The drawing under review shows one solid part. Ordinate dimensions are in mm from its lowest x, y, z. Coordinates: 2 decimals unless noted, no trailing zeros. Write each loop counter-clockwise with the first axis right and the second up, starting at its lowest first coordinate (ties: lowest second). Pieces come first, ordered by that corner, then holes.
1) Add section B-B, the plane y = 1. State the section outline as (x, z) points, then the cut area to 3 significant figures.
2) Add section C-C, the plane z = 0.15. State the section outline as (x, y) points, then the cut area to 3 significant figures.
3) For line 1 (X direction, y = 1.35, z = 0.1); line 2 (X direction, y = 0.6, z = 0.1); line 3 (X direction, y = 0.1, z = 0.1), list the stretches that pass through material, from the lowest coordinate up.
4) Add section A-A, the plane x = 1.5. State the section outline as (y, z) points, then the cut area to 3 significant figures.
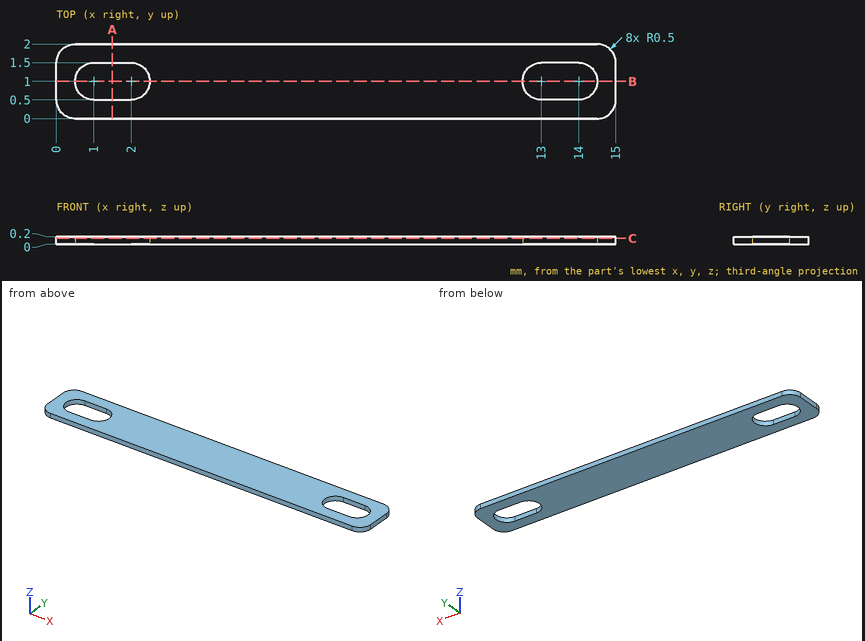
Geometry results:
1. outline: (0, 0) - (0.5, 0) - (0.5, 0.2) - (0, 0.2) - close; (2.5, 0) - (12.5, 0) - (12.5, 0.2) - (2.5, 0.2) - close; (14.5, 0) - (15, 0) - (15, 0.2) - (14.5, 0.2) - close
1. area: 2.20 mm2
2. outline: (0, 0.5) arc R0.5 ccw to (0.5, 0) - (14.5, 0) arc R0.5 ccw to (15, 0.5) - (15, 1.5) arc R0.5 ccw to (14.5, 2) - (0.5, 2) arc R0.5 ccw to (0, 1.5) - close; hole (1, 0.5) - (2, 0.5) arc R0.5 ccw to (2, 1.5) - (1, 1.5) arc R0.5 ccw to start; hole (13, 0.5) - (14, 0.5) arc R0.5 ccw to (14, 1.5) - (13, 1.5) arc R0.5 ccw to start
2. area: 26.2 mm2
3. line 1: x = 0 to 0.64, 2.36 to 12.64, 14.36 to 15
3. line 2: x = 0 to 0.7, 2.3 to 12.7, 14.3 to 15
3. line 3: x = 0.2 to 14.8
4. outline: (0, 0) - (0.5, 0) - (0.5, 0.2) - (0, 0.2) - close; (1.5, 0) - (2, 0) - (2, 0.2) - (1.5, 0.2) - close
4. area: 0.200 mm2
